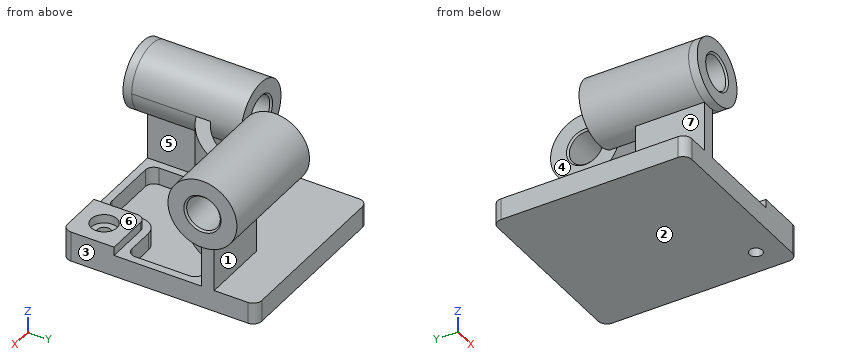
```python
from build123d import *

# Parameters (mm, degrees)
F0_W            = 210
F0_H            = 225
F1_DEPTH        = 25
F3_DEPTH        = 95
F4_R            = 37.5
F5_DEPTH        = 10
F5_DEPTH_BACK   = 127
F6_R            = 40
F7_DEPTH        = 10
F7_DEPTH_BACK   = 127
F8_W            = 60
F8_H            = 60
F9_DEPTH        = 10
F10_R           = 10
F12_DEPTH       = 20
F14_D           = 15
F14_CBORE_D     = 30
F14_CBORE_DEPTH = 10
F15_R           = 10
F16_R           = 19.5
F17_DEPTH       = 235.001
F18_R           = 19.5
F19_DEPTH       = 220.001
F20_SIZE        = 2
F21_R           = 10


with BuildPart() as f1:
    # F0 (on Top) → F1 (new body)
    with BuildSketch(Plane.XY):
        Rectangle(F0_W, F0_H)
    extrude(amount=F1_DEPTH)

    # F2 (on face) → F3 (join)
    with BuildSketch(Plane.XY.offset(25)):
        with BuildLine():
            Line((-71, -32.5), (-71, -112.5))
            Line((-71, -112.5), (-56, -112.5))
            Line((-56, -112.5), (-56, -46.481817))
            ThreePointArc((-56, -46.481817), (7.488853, -14.988853), (38.981817, 48.5))
            Line((38.981817, 48.5), (105, 48.5))
            Line((105, 48.5), (105, 63.5))
            Line((105, 63.5), (25, 63.5))
            ThreePointArc((25, 63.5), (-3.117749, -4.382251), (-71, -32.5))
        make_face()
    extrude(amount=F3_DEPTH)

    # F4 (on face) → F5 (join, two sides)
    with BuildSketch(Plane.XZ.offset(112.5)) as f5_sk:
        with Locations((-63.5, 120)):
            Circle(F4_R)
    extrude(amount=F5_DEPTH)
    extrude(f5_sk.sketch, amount=-F5_DEPTH_BACK)

    # F6 (on face) → F7 (join, two sides)
    with BuildSketch(Plane.YZ.offset(105)) as f7_sk:
        with Locations((56, 120)):
            Circle(F6_R)
    extrude(amount=F7_DEPTH)
    extrude(f7_sk.sketch, amount=-F7_DEPTH_BACK)

    # F8 (on face) → F9 (join)
    with BuildSketch(Plane.XY.offset(25)):
        with Locations((75, -82.5)):
            Rectangle(F8_W, F8_H)
    extrude(amount=F9_DEPTH)

    # F10
    f10_edges = [f1.edges().sort_by_distance(p)[0] for p in [
        (45, -52.5, 30),
    ]]
    fillet(f10_edges, radius=F10_R)

    # F11 (on face) → F12 (cut)
    with BuildSketch(Plane.XY.offset(25)):
        with BuildLine():
            ThreePointArc((46.575508, 39.5), (13.852814, -21.352814), (-47, -54.075508))
            Line((-47, -54.075508), (-47, -103.5))
            Line((-47, -103.5), (36, -103.5))
            Line((36, -103.5), (36, -62.5))
            ThreePointArc((36, -62.5), (41.564971, -49.064971), (55, -43.5))
            Line((55, -43.5), (96, -43.5))
            Line((96, -43.5), (96, 39.5))
            Line((96, 39.5), (46.575508, 39.5))
        make_face()
    extrude(amount=-F12_DEPTH, mode=Mode.SUBTRACT)

    # F14 (through all)
    with Locations(Plane.XY.offset(35)):
        with Locations((75, -82.5)):
            CounterBoreHole(F14_D / 2, F14_CBORE_D / 2, F14_CBORE_DEPTH)

    # F15
    f15_edges = [f1.edges().sort_by_distance(p)[0] for p in [
        (46.575508, 39.5, 15),
        (-47, -54.075508, 15),
        (-47, -103.5, 15),
        (96, 39.5, 15),
        (36, -103.5, 15),
        (96, -43.5, 15),
    ]]
    fillet(f15_edges, radius=F15_R)

    # F16 (on face) → F17 (cut, through all)
    with BuildSketch(Plane.XZ.offset(122.5)):
        with Locations((-63.5, 120)):
            Circle(F16_R)
    extrude(amount=-F17_DEPTH, mode=Mode.SUBTRACT)

    # F18 (on face) → F19 (cut, through all)
    with BuildSketch(Plane.YZ.offset(115)):
        with Locations((56, 120)):
            Circle(F18_R)
    extrude(amount=-F19_DEPTH, mode=Mode.SUBTRACT)

    # F20
    f20_edges = [f1.edges().sort_by_distance(p)[0] for p in [
        (-83, -122.5, 120),
        (115, 36.5, 120),
        (-83, 14.5, 120),
        (-22, 36.5, 120),
    ]]
    chamfer(f20_edges, length=F20_SIZE)

    # F21
    f21_edges = [f1.edges().sort_by_distance(p)[0] for p in [
        (105, -112.5, 17.5),
        (105, 112.5, 12.5),
        (-105, 112.5, 12.5),
        (-105, -112.5, 12.5),
    ]]
    fillet(f21_edges, radius=F21_R)


solid = f1.part
```
Geometry check sheet. Reference: the model listing, model coordinates, mm. Face numbers are marked on the shaded views. A direction names the side the tool comes from. Give positions to 0.01 mm unless a question says otherwise; leave off trailing zeros. Order: outer loops, then holes, each group sorted by start corner. A loop starts at its lowest first (then second) coordinate and runs counter-clockwise, first axis right, second up. Notation, with made-up numbers: (88, 46) - (125, 46) arc R22 cw to (125, 63) - close; hole circle Ø3 at (5.5, -37.75). An arc over 180 degrees is marked (long way). Answer in a Markdown table with one row per item. Add a question column.
Q1. Mould release check, pull along Z, two halves, no side actions. Record for the marked faces 1, 2 and 3: pulls with the +Z half, pulls with the -Z half, needs draft (parallel to the pull), parting line crosses it, or undercut.
Q2. Gauge pin test, flat ends, axial feed: pin 1 (22 mm diameter, centred on x = 75.5, z = 15.5, fed in from -Y); pin 2 (1 mm diameter, centred on x = -7, z = 87.5, fed in from -Y); pin 3 (1 mm diameter, centred on x = 32, y = -96, fed in from +Z). Record the tip position at first contact, or that the pin passes through.
Q3. Tool access check on the marked faces 4, 5, 6 and 7. Record the directions out of +Z, -Z, +X, -X, +Y, -Y that give a thin tool (end or side, any length) a straight path to the whole face; none if there is none.
Q4. Material ranges on probe 1 along Y at (x, z) = (75, 32.75); probe 2 along Z at (x, y) = (35, 65); probe 3 along X at (y, z) = (-64, 10), recorded low to high. Write a range as from..to.
Q5. Cross-section at B-B, the plane y = -8. Enter the section's corners in (x, z), then the cut area to 3 significant figures.
Q6. Cross-section at D-D, the plane x = -63.5. Enter the section's corners in (y, z).
Q7. Cross-section at A-A, the plane x = 75. Enter the section's corners in (y, z), then the cut area to 3 significant figures.
Q8. Cross-section at C-C, the plane z = 147.5. Enter the section's corners in (x, y), then the cut area to 3 significant figures.
Check values:
| question | item | result |
|---|---|---|
| 1 | face 1 | undercut |
| 1 | face 2 | pulls with the -Z half |
| 1 | face 3 | needs draft |
| 2 | pin 1 | stops at y = -112.5 |
| 2 | pin 2 | stops at y = -27.54 |
| 2 | pin 3 | stops at z = 5 |
| 3 | face 4 | +Z, -X, +Y |
| 3 | face 5 | -Y |
| 3 | face 6 | +Z, +X, -Y |
| 3 | face 7 | -X, +Y, -Y |
| 4 | probe 1 | y = -112.5..-97.5, -67.5..-52.5, 48.5..63.5 |
| 4 | probe 2 | z = 0..25, 81.03..102.7, 137.3..158.97 |
| 4 | probe 3 | x = -105..-47, 36..105 |
| 5 | outline | (-105, 0) - (105, 0) - (105, 25) - (96, 25) - (96, 5) - (25.37, 5) - (25.37, 25) - (13.9, 25) - (13.9, 120) - (-6.94, 120) - (-6.94, 25) - (-105, 25) - close; circle Ø75 at (-63.5, 120); hole circle Ø39 at (-63.5, 120) |
| 5 | area | 9,040 mm^2 |
| 6 | outline | (-122.5, 82.5) - (-112.5, 82.5) - (-112.5, 0) - (112.5, 0) - (112.5, 25) - (-32.21, 25) - (-32.21, 82.5) - (14.5, 82.5) - (14.5, 98.5) - (12.5, 100.5) - (-120.5, 100.5) - (-122.5, 98.5) - close; (-122.5, 141.5) - (-120.5, 139.5) - (12.5, 139.5) - (14.5, 141.5) - (14.5, 157.5) - (-122.5, 157.5) - close |
| 7 | outline | (-112.5, 0) - (-90, 0) - (-90, 25) - (-97.5, 25) - (-97.5, 35) - (-112.5, 35) - close; (-75, 0) - (112.5, 0) - (112.5, 25) - (63.5, 25) - (63.5, 80.71) arc R40 ccw (long way) to (48.5, 80.71) - (48.5, 25) - (39.5, 25) - (39.5, 5) - (-43.5, 5) - (-43.5, 25) - (-52.5, 25) - (-52.5, 35) - (-67.5, 35) - (-67.5, 25) - (-75, 25) - close; hole circle Ø39 at (56, 120) |
| 7 | area | 8,550 mm^2 |
| 8 | outline | (-89, -122.5) - (-38, -122.5) - (-38, 14.5) - (-89, 14.5) - close; (-22, 26.95) - (115, 26.95) - (115, 85.05) - (-22, 85.05) - close |
| 8 | area | 14,900 mm^2 |
